Part model, mm, in its own coordinate system. Face numbers are marked on the shaded views. A direction names the side the tool comes from. Give positions to 0.01 mm unless a question says otherwise; leave off trailing zeros. Write each loop counter-clockwise with the first axis right and the second up, starting at its lowest first coordinate (ties: lowest second). Pieces come first, ordered by that corner, then holes. Notation, with made-up numbers: (-39.5, -19.5) - (-3.5, -19.5) arc R7 cw to (-3.5, -13.5) - close; hole circle Ø7 at (42.25, 76). An arc over 180 degrees is marked (long way). Answer in a Markdown table with one row per item. Add a question column.
1. Which spindle directions (+Z, -Z, +X, -X, +Y, -Y) get a long thin tool onto all of the face, cutting with end or side? Do the marked faces 1, 2 and 3. Say none if no direction does.
2. Probe line 1 along X through (y, z) = (2.25, -2) (3 decimals); line 2 along X through (y, z) = (1.25, -0.5). List the from-to ranges inside material, lowest first.
3. Pull direction Z, two halves, no side cores. Call the marked faces 4, 5, 6 and 7: released by +Z, released by -Z, zero draft, split by the parting line, or undercut.
4. Band-saw the part on A-A on x = 0. Write the cut outline in (y, z), plus the area to 3 significant figures.
5. Drop flat-ended pins along their axis: pin 1 Ø1 at (y, z) = (6.5, 2) entering from +X; pin 2 Ø1 at (y, z) = (7.5, 1.5) entering from -X; pin 3 Ø1 at (x, y) = (2, 5.5) entering from -Z; pin 4 Ø3 at (x, y) = (-1, 8) entering from +Z. Give the stop position or say it passes through.
6. Band-saw the part on B-B on y = 5.5. Write the cut outline in (x, z) (3 decimals), plus the area to 3 significant figures.
```python
from build123d import *

# Parameters (mm, degrees)
SKETCH1_W           = 6.2
SKETCH1_H           = 6.2
BOSS_EXTRUDE1_DEPTH = 9
SKETCH2_R           = 5
BOSS_EXTRUDE2_DEPTH = 2
CUT_EXTRUDE1_REACH  = 15.077
CHAMFER1_SIZE       = 2
CHAMFER1_SIZE_2     = 0.932615316


with BuildPart() as part:
    # Sketch1 → Boss-Extrude1 (new body)
    with BuildSketch(Plane(origin=(0, 0, 0), x_dir=(1, 0, 0), z_dir=(0, 1, 0))):
        Rectangle(SKETCH1_W, SKETCH1_H)
    extrude(amount=BOSS_EXTRUDE1_DEPTH)

    # Sketch2 → Boss-Extrude2 (add)
    with BuildSketch(Plane(origin=(0, 9, 0), x_dir=(1, 0, 0), z_dir=(0, 1, 0))):
        with Locations(Location((0, 0, 0), (0, 0, 270))):
            Circle(SKETCH2_R)
    extrude(amount=BOSS_EXTRUDE2_DEPTH)

    # Sketch3 → Cut-Extrude1 (cut, up to next)
    with BuildSketch(Plane(origin=(0, 0, 0), x_dir=(-1, 0, 0), z_dir=(0, -1, 0)), mode=Mode.PRIVATE) as cut_extrude1_sk1:
        with BuildLine():
            ThreePointArc((-1.045, -2.326042777), (0, -2.55), (1.045, -2.326042777))
            Line((1.045, -2.326042777), (1.045, -1.045))
            Line((1.045, -1.045), (-1.045, -1.045))
            Line((-1.045, -1.045), (-1.045, -2.326042777))
        make_face()
    cut_extrude1_tool1 = extrude(cut_extrude1_sk1.sketch, amount=-CUT_EXTRUDE1_REACH, mode=Mode.PRIVATE) & part.part
    # Sketch3 → Cut-Extrude1 (cut, up to next)
    with BuildSketch(Plane(origin=(0, 0, 0), x_dir=(-1, 0, 0), z_dir=(0, -1, 0)), mode=Mode.PRIVATE) as cut_extrude1_sk2:
        with BuildLine():
            Line((1.045, 1.045), (1.045, -1.045))
            Line((1.045, -1.045), (2.326042777, -1.045))
            ThreePointArc((2.326042777, -1.045), (2.493382149, -0.534364538), (2.55, 0))
            ThreePointArc((2.55, 0), (2.493382149, 0.534364538), (2.326042777, 1.045))
            Line((2.326042777, 1.045), (1.045, 1.045))
        make_face()
    cut_extrude1_tool2 = extrude(cut_extrude1_sk2.sketch, amount=-CUT_EXTRUDE1_REACH, mode=Mode.PRIVATE) & part.part
    # Sketch3 → Cut-Extrude1 (cut, up to next)
    with BuildSketch(Plane(origin=(0, 0, 0), x_dir=(-1, 0, 0), z_dir=(0, -1, 0)), mode=Mode.PRIVATE) as cut_extrude1_sk3:
        Polygon((-1.045, -1.045), (1.045, -1.045), (1.045, 1.045), align=None)
    cut_extrude1_tool3 = extrude(cut_extrude1_sk3.sketch, amount=-CUT_EXTRUDE1_REACH, mode=Mode.PRIVATE) & part.part
    # Sketch3 → Cut-Extrude1 (cut, up to next)
    with BuildSketch(Plane(origin=(0, 0, 0), x_dir=(-1, 0, 0), z_dir=(0, -1, 0)), mode=Mode.PRIVATE) as cut_extrude1_sk4:
        Polygon((-1.045, -1.045), (1.045, 1.045), (-1.045, 1.045), align=None)
    cut_extrude1_tool4 = extrude(cut_extrude1_sk4.sketch, amount=-CUT_EXTRUDE1_REACH, mode=Mode.PRIVATE) & part.part
    # Sketch3 → Cut-Extrude1 (cut, up to next)
    with BuildSketch(Plane(origin=(0, 0, 0), x_dir=(-1, 0, 0), z_dir=(0, -1, 0)), mode=Mode.PRIVATE) as cut_extrude1_sk5:
        with BuildLine():
            Line((-2.326042777, -1.045), (-1.045, -1.045))
            Line((-1.045, -1.045), (-1.045, 1.045))
            Line((-1.045, 1.045), (-2.326042777, 1.045))
            ThreePointArc((-2.326042777, 1.045), (-2.55, 0), (-2.326042777, -1.045))
        make_face()
    cut_extrude1_tool5 = extrude(cut_extrude1_sk5.sketch, amount=-CUT_EXTRUDE1_REACH, mode=Mode.PRIVATE) & part.part
    # Sketch3 → Cut-Extrude1 (cut, up to next)
    with BuildSketch(Plane(origin=(0, 0, 0), x_dir=(-1, 0, 0), z_dir=(0, -1, 0)), mode=Mode.PRIVATE) as cut_extrude1_sk6:
        with BuildLine():
            Line((-1.045, 1.045), (1.045, 1.045))
            Line((1.045, 1.045), (1.045, 2.326042777))
            ThreePointArc((1.045, 2.326042777), (0, 2.55), (-1.045, 2.326042777))
            Line((-1.045, 2.326042777), (-1.045, 1.045))
        make_face()
    cut_extrude1_tool6 = extrude(cut_extrude1_sk6.sketch, amount=-CUT_EXTRUDE1_REACH, mode=Mode.PRIVATE) & part.part
    add(cut_extrude1_tool1.solids().sort_by_distance((0, 0, 1.762391))[0], mode=Mode.SUBTRACT)
    add(cut_extrude1_tool2.solids().sort_by_distance((-1.762391, 0, 0))[0], mode=Mode.SUBTRACT)
    add(cut_extrude1_tool3.solids().sort_by_distance((-0.348333, 0, 0.348333))[0], mode=Mode.SUBTRACT)
    add(cut_extrude1_tool4.solids().sort_by_distance((0.348333, 0, -0.348333))[0], mode=Mode.SUBTRACT)
    add(cut_extrude1_tool5.solids().sort_by_distance((1.762391, 0, 0))[0], mode=Mode.SUBTRACT)
    add(cut_extrude1_tool6.solids().sort_by_distance((0, 0, -1.762391))[0], mode=Mode.SUBTRACT)

    # Chamfer1
    # the kernel refuses this chamfer: 2, 0.932615316 mm, written as the material it takes off along each edge
    with BuildSketch(Plane(origin=(0, 11, 0), x_dir=(0, 0, 1), z_dir=(-1, 0, 0))) as chamfer1_piece_1:
        Polygon((5, -CHAMFER1_SIZE), (5 - CHAMFER1_SIZE_2, 0), (5, 0), align=None)
    revolve(axis=Axis((0, 11, 0), (0, 1, 0)), mode=Mode.SUBTRACT)


solid = part.part
```
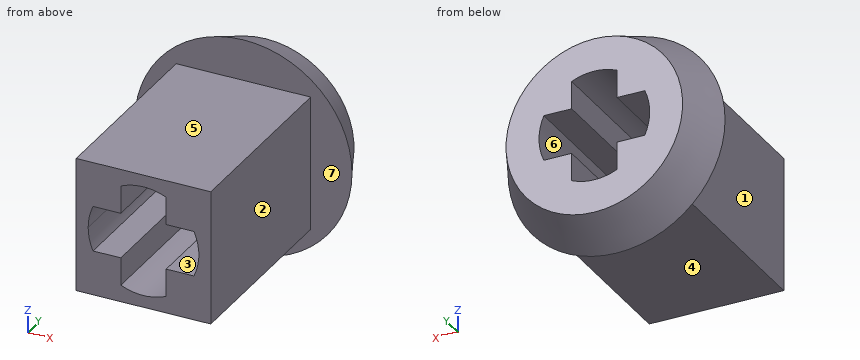
Values:
| question | item | result |
|---|---|---|
| 1 | face 1 | +Z, -Z, -X, -Y |
| 1 | face 2 | +Z, -Z, +X, -Y |
| 1 | face 3 | +Y, -Y |
| 2 | line 1 | x = -3.1 to -1.045, 1.045 to 3.1 |
| 2 | line 2 | x = -3.1 to -2.5, 2.5 to 3.1 |
| 3 | face 4 | released by -Z |
| 3 | face 5 | released by +Z |
| 3 | face 6 | undercut |
| 3 | face 7 | zero draft |
| 4 | outline | (0, -3.1) - (9, -3.1) - (9, -5) - (11, -4.07) - (11, -2.55) - (0, -2.55) - close; (0, 2.55) - (11, 2.55) - (11, 4.07) - (9, 5) - (9, 3.1) - (0, 3.1) - close |
| 4 | area | 17.8 mm² |
| 5 | pin 1 | stops at x = 3.1 |
| 5 | pin 2 | stops at x = -3.1 |
| 5 | pin 3 | stops at z = -3.1 |
| 5 | pin 4 | stops at z = 5 |
| 6 | outline | (-3.1, -3.1) - (3.1, -3.1) - (3.1, 3.1) - (-3.1, 3.1) - close; hole (-2.326, -1.045) - (-1.045, -1.045) - (-1.045, -2.326) arc R2.55 ccw to (1.045, -2.326) - (1.045, -1.045) - (2.326, -1.045) arc R2.55 ccw to (2.326, 1.045) - (1.045, 1.045) - (1.045, 2.326) arc R2.55 ccw to (-1.045, 2.326) - (-1.045, 1.045) - (-2.326, 1.045) arc R2.55 ccw to start |
| 6 | area | 22.1 mm² |
